Part model, mm, in its own coordinate system. A direction names the side the tool comes from. Round coordinates to 2 decimals unless told otherwise and drop trailing zeros. Order: outer loops, then holes, each group sorted by start corner. A loop starts at its lowest first (then second) coordinate and runs counter-clockwise, first axis right, second up. Notation, with made-up numbers: (6.25, -36) -> (54.25, -36) arc R29 ccw to (54.25, -10) -> close; hole circle Ø4 at (3.5, 69). An arc over 180 degrees is marked (long way). Answer as a JSON object with one key per item and string values. Group by question number.
```python
from build123d import *

# Parameters (mm, degrees)
SKETCH029_R     = 13.4
PAD020_DEPTH    = 6
SKETCH030_R     = 11.3
PAD021_DEPTH    = 10
SKETCH031_R     = 9.3
POCKET008_DEPTH = 16.001


with BuildPart() as part:
    # Sketch029 → Pad020 (new body)
    with BuildSketch(Plane.XY):
        with Locations((0, 18)):
            Circle(SKETCH029_R)
    extrude(amount=PAD020_DEPTH)

    # Sketch030 (on Face3 of Pad020) → Pad021 (join)
    with BuildSketch(Plane.XY.offset(6)):
        with Locations((0, 18)):
            Circle(SKETCH030_R)
    extrude(amount=PAD021_DEPTH)

    # Sketch031 (on Face5 of Pad021) → Pocket008 (cut, through all)
    with BuildSketch(Plane.XY.offset(16)):
        with Locations((0, 18)):
            Circle(SKETCH031_R)
    extrude(amount=-POCKET008_DEPTH, mode=Mode.SUBTRACT)


with BuildPart() as part_1:
    # Body038 placement: moved
    add(part.part.moved(Location((0, 0, 4))))


solid = part_1.part
```
Q1. Band-saw the part on C-C (z = 7.75). List the corners of the cut face in (x, y).
Q2. Which spindle directions (+Z, -Z, +X, -X, +Y, -Y) get a long thin tool onto all of the face, cutting with end or side? Do faces 1 (the cylindrical face through (-1.5, 29.2, 14.9)), 2 (the flat face through (9, 21, 4)). Say none if no direction does.
Q3. Two-plate mould, pull along Y, no slides. Class faces 3 (the cylindrical face through (-2.02, 8.92, 12.11)), 4 (the flat face through (-5.9, 10.5, 20)), 5 (the cylindrical face through (-1.744, 31.286, 6.958)): +Y half, -Y half, draft (parallel to the pull), parting line (faces both ways), or undercut.
Q4. Drop flat-ended pins along their axis: pin 1 Ø3 at (x, z) = (3, 6.5) entering from -Y; pin 2 Ø8 at (x, z) = (-9, 6) entering from -Y; pin 3 Ø5 at (x, z) = (-9.5, 17) entering from +Y; pin 4 Ø8 at (x, y) = (-2.5, 18.5) entering from +Z. Give the stop position or say it passes through.
Q5. Wall check: line 1 (Y direction, x = 0, z = 9.75); line 2 (Y direction, x = 0, z = 15.25); line 3 (X direction, y = 17, z = 7.5). Give the ranges that are in metal, low to high. Write a range as [from, to].
Q6. Band-saw the part on A-A (x = 0). List the corners of the cut face in (y, z).
Q7. Band-saw the part on D-D (x = -10.25). List the corners of the cut face in (y, z).
Q8. Band-saw the part on B-B (y = 18). List the corners of the cut face in (x, z).
Completed:
{
 "1": {"outline": "circle Ø26.8 at (0, 18); hole circle Ø18.6 at (0, 18)"},
 "2": {"face 1": "+Z", "face 2": "-Z, +X, -X, +Y, -Y"},
 "3": {"face 3": "undercut", "face 4": "draft", "face 5": "parting line"},
 "4": {"pin 1": "y = 4.68", "pin 2": "y = 5.57", "pin 3": "y = 26.87", "pin 4": "through"},
 "5": {"line 1": "[4.6, 8.7], [27.3, 31.4]", "line 2": "[6.7, 8.7], [27.3, 29.3]", "line 3": "[-13.36, -9.25], [9.25, 13.36]"},
 "6": {"outline": "(4.6, 4) -> (8.7, 4) -> (8.7, 20) -> (6.7, 20) -> (6.7, 10) -> (4.6, 10) -> close; (27.3, 4) -> (31.4, 4) -> (31.4, 10) -> (29.3, 10) -> (29.3, 20) -> (27.3, 20) -> close"},
 "7": {"outline": "(9.37, 4) -> (26.63, 4) -> (26.63, 10) -> (22.76, 10) -> (22.76, 20) -> (13.24, 20) -> (13.24, 10) -> (9.37, 10) -> close"},
 "8": {"outline": "(-13.4, 4) -> (-9.3, 4) -> (-9.3, 20) -> (-11.3, 20) -> (-11.3, 10) -> (-13.4, 10) -> close; (9.3, 4) -> (13.4, 4) -> (13.4, 10) -> (11.3, 10) -> (11.3, 20) -> (9.3, 20) -> close"}
}
